Design review of the part built by this model. Coordinates are the model's own, in mm. A direction names the side the tool comes from. Coordinates: 2 decimals unless noted, no trailing zeros. Write each loop counter-clockwise with the first axis right and the second up, starting at its lowest first coordinate (ties: lowest second). Pieces come first, ordered by that corner, then holes.
Q1. For L1, parallel to Y at x = 9.5, z = 132.05; L2, parallel to Y at x = 19, z = 47.5; L3, parallel to Y at x = 30, z = 131, list the stretches that pass through material, from the lowest coordinate up.
Q2. Take a section at C-C, the plane y = 40. Write out the cut boundary in (x, z), plus the area to 3 significant figures.
Q3. Take a section at B-B, the plane x = 20. Write out the cut boundary in (y, z), plus the area to 3 significant figures.
Q4. The part is to be moulded in two halves that separate along X. For faces 1 (the flat face through (-2, 0, 131)), 2 (the flat face through (20, 0, 134)), 3 (the flat face through (20, -36, 133)), say which applies: released by +X, released by -X, zero draft, split by the parting line, or undercut.
Q5. For faces 4 (the flat face through (20, 6, 129.6)), 5 (the flat face through (20, 46, 87)), 6 (the flat face through (5, 0, 133.5)), list the 3-axis set-ups (+Z, -Z, +X, -X, +Y, -Y) from which the entire face can be reached by the end or side of a thin tool; tool diameter is ignored.
Q6. Take a section at A-A, the plane y = 0. Write out the cut boundary in (x, z), plus the area to 3 significant figures.
Q7. For pin 1 Ø8 at (x, y) = (4, 20.5) entering from -Z; pin 2 Ø4 at (y, z) = (-45.5, 84) entering from +X; pin 3 Ø2 at (x, y) = (30.5, -3.35) entering from -Z; pin 4 Ø4.5 at (x, z) = (28, 131.5) entering from +Y, all flat-tipped, find the tip position at first contact; note any pin that passes through.
Q8. Take a section at D-D, the plane x = 5. Write out the cut boundary in (y, z), plus the area to 3 significant figures.
from build123d import *

# Parameters (mm, degrees)
CROSSBAR_START      = 133
SKETCH_1_W          = 14
SKETCH_1_H          = 116
CROSSBAR_DEPTH      = 12
POST_START          = 43
SKETCH_2_W          = 12
SKETCH_2_H          = 12
POST_DEPTH          = 102
EXTRUDE_START       = 43
SKETCH_3_W          = 12
SKETCH_3_H          = 12
EXTRUDE_3_DEPTH     = 102
CAMERAPLATE_START   = 128
SKETCH_4_W          = 44
SKETCH_4_H          = 44
CAMERAPLATE_DEPTH   = 5.5
CAMERARECESS_START  = 128
SKETCH_5_W          = 25.6
SKETCH_5_H          = 24.3
CAMERARECESS_DEPTH  = 1.6
LENSWINDOW_START    = 127
SKETCH_6_R          = 5
LENSWINDOW_DEPTH    = 7
CAMSCREW_START      = 127
SKETCH_7_R          = 0.9
CAMSCREW_DEPTH      = 7
CUT_EXTRUDE_START   = 127
SKETCH_8_R          = 0.9
CUT_EXTRUDE_4_DEPTH = 7
SKETCH_9_R          = 0.9
CUT_EXTRUDE_5_DEPTH = 7
SKETCH_10_R         = 0.9
CUT_EXTRUDE_6_DEPTH = 7


with BuildPart() as part:
    # 草图1 → Crossbar (new body)
    with BuildSketch(Plane.XY.offset(CROSSBAR_START)):
        with Locations((20, 0)):
            Rectangle(SKETCH_1_W, SKETCH_1_H)
    extrude(amount=CROSSBAR_DEPTH)

    # 草图2 → Post (add)
    with BuildSketch(Plane.XY.offset(POST_START)):
        with Locations((20, -52)):
            Rectangle(SKETCH_2_W, SKETCH_2_H)
    extrude(amount=POST_DEPTH)

    # 草图3 → 凸台-拉伸3 (add)
    with BuildSketch(Plane.XY.offset(EXTRUDE_START)):
        with Locations((20, 52)):
            Rectangle(SKETCH_3_W, SKETCH_3_H)
    extrude(amount=EXTRUDE_3_DEPTH)

    # 草图4 → CameraPlate (add)
    with BuildSketch(Plane.XY.offset(CAMERAPLATE_START)):
        with Locations((20, 0)):
            Rectangle(SKETCH_4_W, SKETCH_4_H)
    extrude(amount=CAMERAPLATE_DEPTH)

    # 草图5 → CameraRecess (cut)
    with BuildSketch(Plane.XY.offset(CAMERARECESS_START)):
        with Locations((20, 2.9)):
            Rectangle(SKETCH_5_W, SKETCH_5_H)
    extrude(amount=CAMERARECESS_DEPTH, mode=Mode.SUBTRACT)

    # 草图6 → LensWindow (cut)
    with BuildSketch(Plane.XY.offset(LENSWINDOW_START)):
        with Locations(Location((20, 0, 0), (0, 0, 180))):
            Circle(SKETCH_6_R)
    extrude(amount=LENSWINDOW_DEPTH, mode=Mode.SUBTRACT)

    # 草图7 → CamScrew (cut)
    with BuildSketch(Plane.XY.offset(CAMSCREW_START)):
        with Locations(Location((9.5, -3.35, 0), (0, 0, 180))):
            Circle(SKETCH_7_R)
    extrude(amount=CAMSCREW_DEPTH, mode=Mode.SUBTRACT)

    # 草图8 → 切除-拉伸4 (cut)
    with BuildSketch(Plane.XY.offset(CUT_EXTRUDE_START)):
        with Locations(Location((9.5, 9.15, 0), (0, 0, 180))):
            Circle(SKETCH_8_R)
    extrude(amount=CUT_EXTRUDE_4_DEPTH, mode=Mode.SUBTRACT)

    # 草图9 → 切除-拉伸5 (cut)
    with BuildSketch(Plane.XY.offset(CUT_EXTRUDE_START)):
        with Locations(Location((30.5, -3.35, 0), (0, 0, 180))):
            Circle(SKETCH_9_R)
    extrude(amount=CUT_EXTRUDE_5_DEPTH, mode=Mode.SUBTRACT)

    # 草图10 → 切除-拉伸6 (cut)
    with BuildSketch(Plane.XY.offset(CUT_EXTRUDE_START)):
        with Locations(Location((30.5, 9.15, 0), (0, 0, 180))):
            Circle(SKETCH_10_R)
    extrude(amount=CUT_EXTRUDE_6_DEPTH, mode=Mode.SUBTRACT)


solid = part.part
Responses:
1. L1: y = -22 to -4.25, -2.45 to 8.25, 10.05 to 22
1. L2: y = -58 to -46, 46 to 58
1. L3: y = -22 to -4.1, -2.6 to 8.4, 9.9 to 22
2. outline: (13, 133) - (27, 133) - (27, 145) - (13, 145) - close
2. area: 168 mm2
3. outline: (-58, 43) - (-46, 43) - (-46, 133) - (-22, 133) - (-22, 128) - (-9.25, 128) - (-9.25, 129.6) - (-5, 129.6) - (-5, 134) - (5, 134) - (5, 129.6) - (15.05, 129.6) - (15.05, 128) - (22, 128) - (22, 133) - (46, 133) - (46, 43) - (58, 43) - (58, 145) - (-58, 145) - close
3. area: 3,690 mm2
4. face 1: released by -X
4. face 2: undercut
4. face 3: zero draft
5. face 4: -Z
5. face 5: -Z, +X, -X
5. face 6: +Z, -X, +Y, -Y
6. outline: (-2, 128) - (7.2, 128) - (7.2, 129.6) - (15, 129.6) - (15, 134) - (25, 134) - (25, 129.6) - (32.8, 129.6) - (32.8, 128) - (42, 128) - (42, 133.5) - (27, 133.5) - (27, 145) - (13, 145) - (13, 133.5) - (-2, 133.5) - close
6. area: 318 mm2
7. pin 1: stops at z = 128
7. pin 2: stops at x = 26
7. pin 3: stops at z = 129.6
7. pin 4: stops at y = 58
8. outline: (-22, 128) - (22, 128) - (22, 133.5) - (-22, 133.5) - close
8. area: 242 mm2
